The listing builds one solid part. Answer for the finished solid, in the listing's coordinates (mm). A direction names the side the tool comes from. Coordinates: 2 decimals unless noted, no trailing zeros. Write each loop counter-clockwise with the first axis right and the second up, starting at its lowest first coordinate (ties: lowest second). Pieces come first, ordered by that corner, then holes. Notation, with made-up numbers: M 70,79.25 L 84,79.25 A26 ccw 84,118.25 Z; hole C 46.25,-2.75 d11. An arc over 180 degrees is marked long. Write item = value, one per line. Start each with the question number.
```python
from build123d import *

# Parameters (mm, degrees)
BOSS_EXTRUDE1_DEPTH                             = 6.54
BOSS_EXTRUDE4_DEPTH                             = 27.000000000000004
CSK_FOR_M3_FLAT_HEAD_MACHINE_SCREW2_D           = 4.93
CSK_FOR_M3_FLAT_HEAD_MACHINE_SCREW2_CSINK_D     = 12
CSK_FOR_M3_FLAT_HEAD_MACHINE_SCREW2_CSINK_ANGLE = 90
BOSS_EXTRUDE5_DEPTH                             = 20
BOSS_EXTRUDE6_DEPTH                             = 28.999999999999996
CUT_EXTRUDE1_REACH                              = 86.042
SKETCH18_RX                                     = 21.5
SKETCH18_RY                                     = 11.999999999999996
CUT_EXTRUDE2_REACH                              = 89.09
CUT_EXTRUDE3_DEPTH                              = 8.999999999999996
CUT_EXTRUDE4_DEPTH                              = 8.999999999999996
CSK_FOR_M3_FLAT_HEAD_MACHINE_SCREW4_D           = 4.93
CSK_FOR_M3_FLAT_HEAD_MACHINE_SCREW4_DEPTH       = 6.54
CSK_FOR_M3_FLAT_HEAD_MACHINE_SCREW4_CSINK_D     = 12
CSK_FOR_M3_FLAT_HEAD_MACHINE_SCREW4_CSINK_ANGLE = 90
CSK_FOR_M3_FLAT_HEAD_MACHINE_SCREW5_D           = 4.93
CSK_FOR_M3_FLAT_HEAD_MACHINE_SCREW5_CSINK_D     = 12
CSK_FOR_M3_FLAT_HEAD_MACHINE_SCREW5_CSINK_ANGLE = 90


with BuildPart() as part:
    # Sketch1 → Boss-Extrude1 (new body)
    with BuildSketch(Plane.XY):
        Polygon((-30.000000000000004, 59.99999999999999), (29.999999999999996, 59.99999999999999), (30.00000000000001, -60.00000000000001), (-29.99999999999999, -60.00000000000001), align=None)
    extrude(amount=BOSS_EXTRUDE1_DEPTH)

    # Sketch7 → Boss-Extrude4 (add)
    with BuildSketch(Plane.XY.offset(6.54)):
        with BuildLine():
            Line((-30.000000000000004, 44.48331477354787), (-30.000000000000004, 29.516685226452115))
            ThreePointArc((-30.000000000000004, 29.516685226452115), (-15.999999999999986, 36.99999999999999), (-30.000000000000004, 44.48331477354787))
        make_face()
    extrude(amount=BOSS_EXTRUDE4_DEPTH)

    # CSK for M3 Flat Head Machine Screw2 (through all)
    with Locations(Plane(origin=(-10, -40, 6.54), x_dir=(1, 0, 0), z_dir=(0, 0, 1))):
        with Locations((0, 0), (20, 0), (0, 80), (20, 80)):
            CounterSinkHole(CSK_FOR_M3_FLAT_HEAD_MACHINE_SCREW2_D / 2, CSK_FOR_M3_FLAT_HEAD_MACHINE_SCREW2_CSINK_D / 2, counter_sink_angle=CSK_FOR_M3_FLAT_HEAD_MACHINE_SCREW2_CSINK_ANGLE)

    # Sketch10 → Boss-Extrude5 (add)
    with BuildSketch(Plane(origin=(0, 0, 0), x_dir=(-1, 0, 0), z_dir=(0, 0, -1))):
        Polygon((20, 20), (26.540000000000003, 20), (26.540000000000006, -20.000000000000007), (20, -20.000000000000007), align=None)
        Polygon((-20, -20), (-20, 19.999999999999993), (-26.540000000000003, 19.999999999999993), (-26.54, -20), align=None)
    extrude(amount=BOSS_EXTRUDE5_DEPTH)

    # Sketch17 → Boss-Extrude6 (add)
    with BuildSketch(Plane.XY.offset(6.54)):
        Polygon((-30, 9.999999999999995), (30.000000000000014, 9.999999999999995), (30.00000000000001, -30.000000000000007), (-29.999999999999996, -30.000000000000007), align=None)
    extrude(amount=BOSS_EXTRUDE6_DEPTH)

    # Sketch18 → Cut-Extrude1 (cut, up to next)
    with BuildSketch(Plane(origin=(0, 9.999999999999995, 0), x_dir=(1, 0, 0), z_dir=(0, 1, 0)), mode=Mode.PRIVATE) as cut_extrude1_sk1:
        with Locations((5.500000000000008, -20.091951128620167)):
            Ellipse(SKETCH18_RX, SKETCH18_RY)
    cut_extrude1_tool1 = extrude(cut_extrude1_sk1.sketch, amount=-CUT_EXTRUDE1_REACH, mode=Mode.PRIVATE) & part.part
    add(cut_extrude1_tool1.solids().sort_by_distance((5.5, 10, 20.091951))[0], mode=Mode.SUBTRACT)

    # Sketch21 → Cut-Extrude2 (cut, up to next)
    with BuildSketch(Plane.XY.offset(35.53999999999999), mode=Mode.PRIVATE) as cut_extrude2_sk1:
        Polygon((-15.99999999999999, 9.999999999999995), (27.00000000000001, 9.999999999999995), (27.00000000000002, -30.000000000000007), (-15.999999999999986, -30.000000000000007), align=None)
    cut_extrude2_tool1 = extrude(cut_extrude2_sk1.sketch, amount=-CUT_EXTRUDE2_REACH, mode=Mode.PRIVATE) & part.part
    add(cut_extrude2_tool1.solids().sort_by_distance((5.5, -10, 35.54))[0], mode=Mode.SUBTRACT)

    # Sketch23 → Cut-Extrude3 (cut)
    with BuildSketch(Plane(origin=(-15.99999999999999, -1.39e-15, 0), x_dir=(0, 0, -1), z_dir=(1, 9e-17, 0))):
        Polygon((-34.139999999999986, 7.9999999999999964), (-32.13999999999999, 7.9999999999999964), (-32.139999999999986, -28.000000000000007), (-34.139999999999986, -28), align=None)
    extrude(amount=-CUT_EXTRUDE3_DEPTH, mode=Mode.SUBTRACT)

    # Sketch24 → Cut-Extrude4 (cut)
    with BuildSketch(Plane.ZY.offset(-27.000000000000014)):
        Polygon((32.13999999999999, 7.9999999999999885), (34.14, 7.9999999999999885), (34.14, -28.00000000000001), (32.14, -28.00000000000001), align=None)
    extrude(amount=-CUT_EXTRUDE4_DEPTH, mode=Mode.SUBTRACT)

    # CSK for M3 Flat Head Machine Screw4
    with Locations(Plane(origin=(-26.54, 0, -10), x_dir=(0, -1, 0), z_dir=(-1, 0, 0))):
        with Locations((0, 0)):
            CounterSinkHole(CSK_FOR_M3_FLAT_HEAD_MACHINE_SCREW4_D / 2, CSK_FOR_M3_FLAT_HEAD_MACHINE_SCREW4_CSINK_D / 2, depth=CSK_FOR_M3_FLAT_HEAD_MACHINE_SCREW4_DEPTH, counter_sink_angle=CSK_FOR_M3_FLAT_HEAD_MACHINE_SCREW4_CSINK_ANGLE)

    # CSK for M3 Flat Head Machine Screw5 (through all)
    with Locations(Plane(origin=(26.54, 0, -10), x_dir=(0, 1, 0), z_dir=(1, 0, 0))):
        with Locations((0, 0)):
            CounterSinkHole(CSK_FOR_M3_FLAT_HEAD_MACHINE_SCREW5_D / 2, CSK_FOR_M3_FLAT_HEAD_MACHINE_SCREW5_CSINK_D / 2, counter_sink_angle=CSK_FOR_M3_FLAT_HEAD_MACHINE_SCREW5_CSINK_ANGLE)


solid = part.part
```
1. The part is cut by section B-B, the plane z = -10. Write down the section's boundary in (x, y) (3 decimals).
2. The part is cut by section C-C, the plane y = 40. Write down the section's boundary in (x, z) (3 decimals), and give its area (3 significant figures).
3. For a pull along Y with two mould halves and no side action, classify faces 1 (the face through (23, -20, -10)), 2 (the face through (0, 60, 3)), 3 (the face through (10.572, -42.574, 3.177)) as pulls with the +Y half, pulls with the -Y half, needs draft (parallel to the pull), parting line crosses it, or undercut.
4. The part is cut by section D-D, the plane z = 27.5. Write down the section's boundary in (x, y), and give its area (3 significant figures).
5. For faces 4 (the face through (-20, -10, 34.14)), 5 (the face through (-6, -30, 8)), 6 (the face through (20, 4, -10)), 7 (the face through (26.54, 5, -5)), determine the directions among +Z, -Z, +X, -X, +Y, -Y from which every point of the face is accessible in a straight line to the end or side of a thin tool.
6. Straight lines are drawn through the part: L1, parallel to Y at x = -10, z = 2 (3 decimals); L2, parallel to X at y = 40, z = 0.8 (3 decimals); L3, parallel to X at y = 5, z = 21. For each, find the intervals that lie inside material, in ascending order. Write a range as [from, to].
7. Each of these flat-tipped pins is pushed along its axis until it touches: pin 1 (10 mm diameter, centred on y = 10, z = -6.5, fed in from -X); pin 2 (12 mm diameter, centred on x = -7.5, y = 15, fed in from +Z); pin 3 (1 mm diameter, centred on x = -21.5, z = 33, fed in from -Y). Where does it stop, or does it pass through?
8. The part is cut by section A-A, the plane z = -2. Write down the section's boundary in (x, y).
Solution:
q1.outline = M -26.54,-20 L -20,-20 L -20,-2.465 L -23.005,-2.465 L -26.54,-6 Z; M -26.54,6 L -23.005,2.465 L -20,2.465 L -20,20 L -26.54,20 Z; M 20,-20 L 26.54,-20 L 26.54,-6 L 23.005,-2.465 L 20,-2.465 Z; M 20,2.465 L 23.005,2.465 L 26.54,6 L 26.54,20 L 20,20 Z
q2.outline = M -30,0 L -12.465,0 L -12.465,3.005 L -16,6.54 L -16.515,6.54 L -16.515,33.54 L -30,33.54 Z; M -7.535,0 L 7.535,0 L 7.535,3.005 L 4,6.54 L -4,6.54 L -7.535,3.005 Z; M 12.465,0 L 30,0 L 30,6.54 L 16,6.54 L 12.465,3.005 Z
q2.area = 667 mm^2
q3.face_1 = pulls with the -Y half
q3.face_2 = pulls with the +Y half
q3.face_3 = undercut
q4.outline = M -30,-30 L -16,-30 L -16,10 L -30,10 Z; M -30,29.52 A9 ccw long -30,44.48 Z; M 27,-30 L 30,-30 L 30,10 L 27,10 Z
q4.area = 892 mm^2
q5.face_4 = +X
q5.face_5 = +Z, +X, -X, -Y
q5.face_6 = -Z, +Y, -Y
q5.face_7 = -Z, +X, +Y, -Y
q6.L1 = [-60, -42.465], [-37.535, 37.535], [42.465, 60]
q6.L2 = [-30, -12.465], [-7.535, 7.535], [12.465, 30]
q6.L3 = [-30, -16], [27, 30]
q7.pin_1 = -26.54
q7.pin_2 = 12.28
q7.pin_3 = -30
q8.outline = M -26.54,-20 L -20,-20 L -20,20 L -26.54,20 Z; M 20,-20 L 26.54,-20 L 26.54,20 L 20,20 Z
